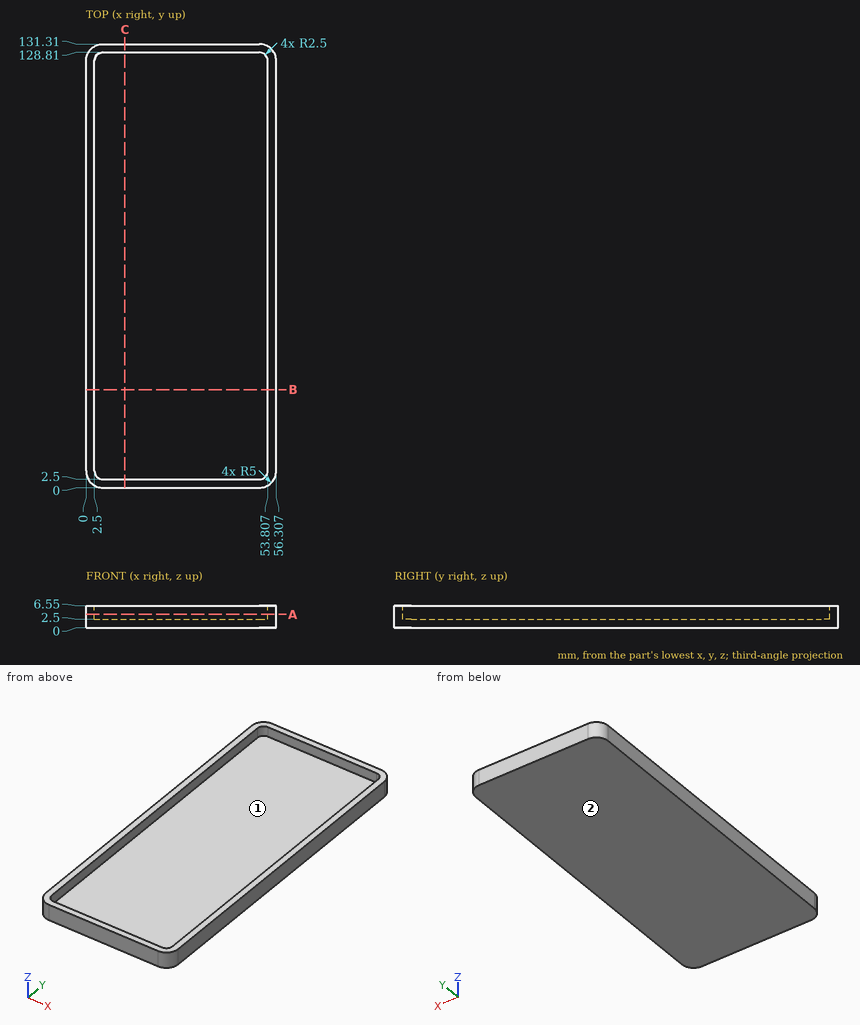
Design review of the part shown in the three views and the two pictorial views. Dimensions are in mm from the part's minimum x, y and z. Coordinates: 2 decimals unless noted, no trailing zeros. Write each loop counter-clockwise with the first axis right and the second up, starting at its lowest first coordinate (ties: lowest second). Pieces come first, ordered by that corner, then holes.
(1) Add section C-C on x = 11.5. Give the boundary of the cut face in (y, z).
(2) Add section B-B on y = 29. Give the boundary of the cut face in (x, z), then the cut area to 3 significant figures.
(3) For pin 1 Ø12 at (x, y) = (47, 43.5) entering from +Z, flat-tipped, find the tip position at first contact; note if it passes through.
(4) Wall thickness on probe 1 along X at (y, z) = (70.5, 2.75); probe 2 along Y at (x, z) = (51, 3.75); probe 3 along Z at (x, y) = (40, 107.5): over which ranges is each line inside the solid? List them lowest first.
(5) The part is to be moulded in two halves that separate along X. For the marked faces 1 and 2, say which applies: +X half, -X half, draft (parallel to the pull), parting line (faces both ways), or undercut.
(6) Add section A-A on z = 4. Give the boundary of the cut face in (x, y).
Answer sheet:
1. outline: (0, 0) - (131.31, 0) - (131.31, 6.55) - (128.81, 6.55) - (128.81, 2.5) - (2.5, 2.5) - (2.5, 6.55) - (0, 6.55) - close
2. outline: (0, 0) - (56.31, 0) - (56.31, 6.55) - (53.81, 6.55) - (53.81, 2.5) - (2.5, 2.5) - (2.5, 6.55) - (0, 6.55) - close
2. area: 161 mm2
3. pin 1: stops at z = 2.5
4. probe 1: x = 0 to 2.5, 53.81 to 56.31
4. probe 2: y = 0 to 2.5, 128.81 to 131.31
4. probe 3: z = 0 to 2.5
5. face 1: undercut
5. face 2: draft
6. outline: (0, 5) arc R5 ccw to (5, 0) - (51.31, 0) arc R5 ccw to (56.31, 5) - (56.31, 126.31) arc R5 ccw to (51.31, 131.31) - (5, 131.31) arc R5 ccw to (0, 126.31) - close; hole (2.5, 5) arc R2.5 ccw to (5, 2.5) - (51.31, 2.5) arc R2.5 ccw to (53.81, 5) - (53.81, 126.31) arc R2.5 ccw to (51.31, 128.81) - (5, 128.81) arc R2.5 ccw to (2.5, 126.31) - close
